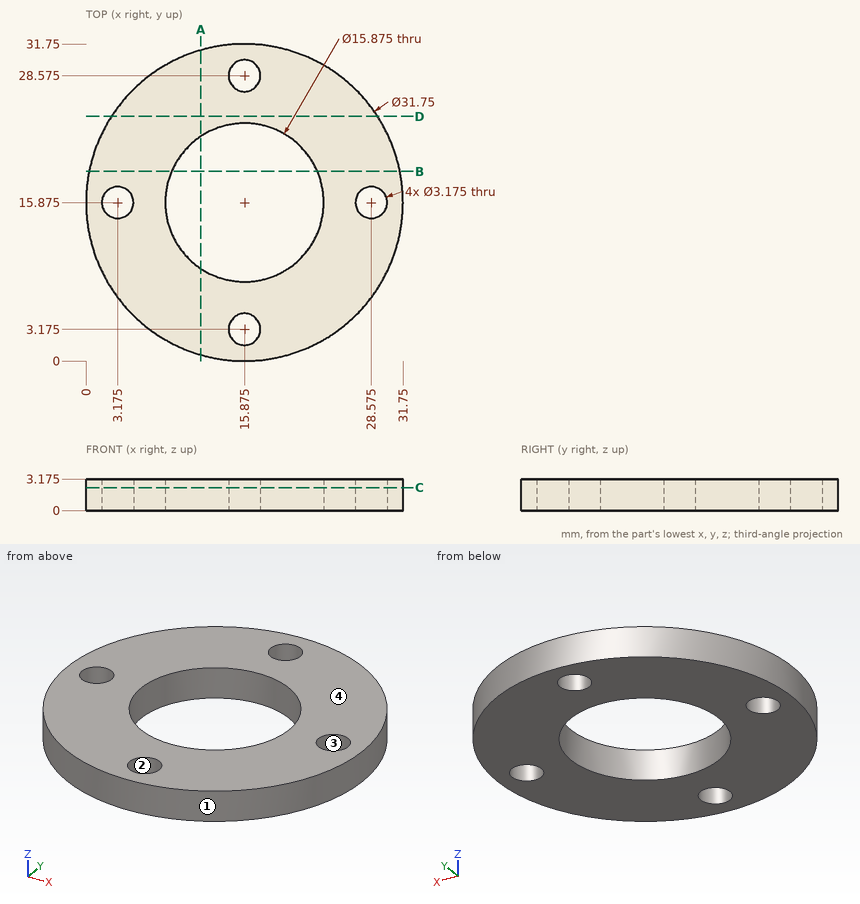
Design review of the part shown in the three views and the two pictorial views. Dimensions are in mm from the part's minimum x, y and z. Round coordinates to 2 decimals unless told otherwise and drop trailing zeros. Order: outer loops, then holes, each group sorted by start corner. A loop starts at its lowest first (then second) coordinate and runs counter-clockwise, first axis right, second up. Notation, with made-up numbers: (36, 59) - (81, 59) arc R8 cw to (81, 73) - close; hole circle Ø5 at (-2, 57.5). An arc over 180 degrees is marked (long way). One line per question, with ' | ' between items.
Item 1: Take a section at D-D, the plane y = 24.5. Write out the cut boundary in (x, z) (3 decimals), then the cut area to 3 significant figures.
Checks:
outline: (2.547, 0) - (29.203, 0) - (29.203, 3.175) - (2.547, 3.175) - close | area: 84.6 mm²
Item 2: For P1, Ø1.5, axis at y = 18.5, z = 0.5, coming from the +X side; P2, Ø2.5, axis at x = 28.575, y = 15.875, coming from the -Z side; P3, Ø1.5, axis at y = 7, z = 0.5, coming from the -X side, all flat-tipped, find the tip position at first contact; note any pin that passes through.
Checks:
P1: x = 31.64 | P2: through | P3: x = 2.24
Item 3: Take a section at B-B, the plane y = 19. Write out the cut boundary in (x, z) (3 decimals), then the cut area to 3 significant figures.
Checks:
outline: (0.311, 0) - (8.579, 0) - (8.579, 3.175) - (0.311, 3.175) - close; (23.171, 0) - (31.439, 0) - (31.439, 3.175) - (23.171, 3.175) - close | area: 52.5 mm²
Item 4: Wall thickness on line 1 (Y direction, x = 16, z = 0.7); line 2 (X direction, y = 14, z = 0.9); line 3 (X direction, y = 4, z = 1.35): over which ranges is each line inside the solid? List them lowest first. Write a range as [from, to].
Checks:
line 1: [0, 1.59], [4.76, 7.94], [23.81, 26.99], [30.16, 31.75] | line 2: [0.11, 8.16], [23.59, 31.64] | line 3: [5.34, 14.52], [17.23, 26.41]
Item 5: Take a section at C-C, the plane z = 2.3. Give the number of separate pieces and of enclosed holes in the cut face, then the cut area to 3 significant figures.
Checks:
separate pieces: 1 | enclosed holes: 5 | area: 562 mm²
Item 6: Take a section at A-A, the plane x = 11.5. Write out the cut boundary in (y, z) (3 decimals).
Checks:
outline: (0.615, 0) - (9.252, 0) - (9.252, 3.175) - (0.615, 3.175) - close; (22.498, 0) - (31.135, 0) - (31.135, 3.175) - (22.498, 3.175) - close
Item 7: Draft analysis for pull direction X (two halves, no side actions). For the marked faces 1, 2, 3 and 4, state which applies: +X half, -X half, draft (parallel to the pull), parting line (faces both ways), or undercut.
Checks:
face 1: parting line | face 2: undercut | face 3: undercut | face 4: draft
